```python
from build123d import *

# Parameters (mm, degrees)
BOSS_EXTRUDE1_DEPTH = 500
CUT_EXTRUDE1_DEPTH  = 497
SKETCH3_R           = 4
CUT_EXTRUDE2_DEPTH  = 497
SKETCH4_R           = 2.75
CUT_EXTRUDE3_DEPTH  = 5


with BuildPart() as part:
    # Sketch1 → Boss-Extrude1 (new body)
    with BuildSketch(Plane.XY):
        with BuildLine():
            Line((0, 0), (175, 0))
            Line((175, 0), (175, 137.5))
            ThreePointArc((175, 137.5), (87.5, 225), (0, 137.5))
            Line((0, 137.5), (0, 0))
        make_face()
    extrude(amount=BOSS_EXTRUDE1_DEPTH)

    # Sketch2 → Cut-Extrude1 (cut)
    with BuildSketch(Plane.XY.offset(500)):
        with BuildLine():
            Line((172.61875, 2.38125), (172.61875, 137.5))
            ThreePointArc((172.61875, 137.5), (87.5, 222.61875), (2.38125, 137.5))
            Line((2.38125, 137.5), (2.38125, 2.38125))
            Line((2.38125, 2.38125), (172.61875, 2.38125))
        make_face()
    extrude(amount=-CUT_EXTRUDE1_DEPTH, mode=Mode.SUBTRACT)

    # Sketch3 → Cut-Extrude2 (cut)
    with BuildSketch(Plane(origin=(175, 0, 0), x_dir=(0, 0, -1), z_dir=(1, 0, 0))):
        with Locations((-490, 10)):
            Circle(SKETCH3_R)
    extrude(amount=-CUT_EXTRUDE2_DEPTH, mode=Mode.SUBTRACT)

    # Sketch4 → Cut-Extrude3 (cut)
    with BuildSketch(Plane(origin=(0, 225, 0), x_dir=(1, 0, 0), z_dir=(0, 1, 0))):
        with Locations((87.5, -70)):
            Circle(SKETCH4_R)
    extrude(amount=-CUT_EXTRUDE3_DEPTH, mode=Mode.SUBTRACT)


solid = part.part
```
The model under review builds one solid part; all positions refer to its coordinate system, in mm. A direction names the side the tool comes from. Round coordinates to 2 decimals unless told otherwise and drop trailing zeros. Order: outer loops, then holes, each group sorted by start corner. A loop starts at its lowest first (then second) coordinate and runs counter-clockwise, first axis right, second up. Notation, with made-up numbers: (82.25, 79) -> (102.25, 79) arc R31 ccw to (102.25, 107) -> close; hole circle Ø1 at (3.5, 32.25). An arc over 180 degrees is marked (long way). One line per item, written item: value. Start each with the question number.
Q1. Take a section at C-C (x = 78). Write out the cut boundary in (y, z).
Q2. Machinability: for faces 5 (the face through (86, 114, 3)), 6 (the face through (86, 114, 0)), which of the approach directions +Z, -Z, +X, -X, +Y, -Y give a long, thin tool a straight path to every point of the face, cutting with its end or side? Answer none if there is none.
Q3. Mouldability with a two-part tool opening along Y and no side actions: class faces 1 (the face through (86, 0, 246)), 2 (the face through (2.381, 71, 255)), 3 (the face through (89.42, 224.98, 246.5)), 4 (the face through (0, 70, 246)) as released by +Y, released by -Y, zero draft, split by the parting line, or undercut.
Q4. Clearance check with flat-ended pins moving along their axes: pin 1 Ø1.5 at (x, z) = (126, 306.5) entering from +Y; pin 2 Ø8 at (y, z) = (189, 254.5) entering from +X; pin 3 Ø5 at (x, z) = (87.5, 70) entering from +Y. State where each tip first meets the part, or that it passes through.
Q5. Take a section at A-A (z = 331.5). Write out the cut boundary in (x, y), and give its area (3 significant figures).
Q6. Wall thickness on line 1 (X direction, y = 120.5, z = 125); line 2 (Z direction, x = 87.5, y = 223.15); line 3 (X direction, y = 141, z = 305.5): over which ranges is each line inside the solid? List them lowest first.
Q7. Take a section at B-B (y = 123). Write out the cut boundary in (x, z), and give its area (3 significant figures).
Reported:
1. outline: (0, 0) -> (224.48, 0) -> (224.48, 500) -> (222.09, 500) -> (222.09, 3) -> (2.38, 3) -> (2.38, 500) -> (0, 500) -> close
2. face 5: +Z
2. face 6: -Z, +X, -X, +Y, -Y
3. face 1: released by -Y
3. face 2: undercut
3. face 3: released by +Y
3. face 4: zero draft
4. pin 1: stops at y = 216.44
4. pin 2: stops at x = 160.98
4. pin 3: stops at y = 2.38
5. outline: (0, 0) -> (175, 0) -> (175, 137.5) arc R87.5 ccw to (0, 137.5) -> close; hole (2.38, 2.38) -> (172.62, 2.38) -> (172.62, 137.5) arc R85.12 ccw to (2.38, 137.5) -> close
5. area: 1,710 mm2
6. line 1: x = 0 to 2.38, 172.62 to 175
6. line 2: z = 0 to 67.25, 72.75 to 500
6. line 3: x = 0.07 to 2.45, 172.55 to 174.93
7. outline: (0, 0) -> (175, 0) -> (175, 500) -> (172.62, 500) -> (172.62, 3) -> (2.38, 3) -> (2.38, 500) -> (0, 500) -> close
7. area: 2,890 mm2
